Here's how the part is built. I have some questions about the finished solid (model axes, mm). A direction names the side the tool comes from. Coordinates: 2 decimals unless noted, no trailing zeros. Loops run counter-clockwise (first coordinate to the right, second up) from the corner with the lowest first, then second, coordinate; pieces in that order, holes last. Notation, with made-up numbers: (23, -11.75) -> (46, -11.75) arc R18 ccw to (46, 22.25) -> close; hole circle Ø4 at (44.5, 35.25). An arc over 180 degrees is marked (long way). Answer as a JSON object with one key per item and string values. Group by question number.
Q1. I want a section at B-B on x = -1.75. Write out the boundary of the cut face in (y, z), then the cut area to 3 significant figures.
Q2. I need wall thicknesses on line 1 (Z direction, x = -4, y = -11.5); line 2 (Z direction, x = 7, y = -13.5) (3 decimals); line 3 (Y direction, x = 2.75, z = -12.7). Which ranges of each line are inside material? Lowest first, please.
Q3. Thinking about a two-plate mould opening in Y: for faces 1 (the cylindrical face through (0.13, -13.64, -13.88)), 2 (the flat face through (12.7, 21, -20)), 3 (the flat face through (0, -19.05, -25)), which applies, released by +Y, released by -Y, zero draft, split by the parting line, or undercut?
Q4. I want a section at D-D on y = 27.5. Write out the boundary of the cut face in (x, z).
Q5. I want a section at C-C on z = -45. Write out the boundary of the cut face in (x, y).
Q6. I want a section at A-A on z = -12.7. Write out the boundary of the cut face in (x, y), then the cut area to 3 significant figures.
Q7. On a 3-axis mill with a long thin cutter (end or side, diameter ignored), from which of +Z, -Z, +X, -X, +Y, -Y can I reach the whole of each face in a straight line? I mean faces 4 (the flat face through (-11, 0, -26)), 5 (the flat face through (-9.144, -9, -26)), 6 (the flat face through (0, -9, -47.244)). Say none if no direction works.
Q8. I'm going to push flat-ended pins straight in: pin 1 (12 mm diameter, centred on x = -3.5, y = 38, fed in from -Z); pin 2 (8 mm diameter, centred on x = 3, y = -8, fed in from +Z); pin 3 (5.5 mm diameter, centred on y = -9, z = -18, fed in from -X). Where does each tip first touch, or does it pass through?
```python
from build123d import *

# Parameters (mm, degrees)
BOSS_EXTRUDE1_DEPTH = 12.7
SKETCH2_W           = 18.288
SKETCH2_H           = 43.688
BOSS_EXTRUDE2_DEPTH = 19.05
SKETCH3_R           = 2.5527
CUT_EXTRUDE1_DEPTH  = 22.844
CHAMFER1_SIZE       = 1


with BuildPart() as part:
    # Sketch1 → Boss-Extrude1 (new body, symmetric)
    with BuildSketch(Plane(origin=(0, 0, 0), x_dir=(0, 0, -1), z_dir=(1, 0, 0))):
        Polygon((0, 0), (0, 77.724), (50.8, 5.174081258), (50.8, 0), align=None)
    extrude(amount=BOSS_EXTRUDE1_DEPTH, both=True)

    # Sketch2 → Boss-Extrude2 (add)
    with BuildSketch(Plane.XZ):
        with Locations((0, -25.4)):
            Rectangle(SKETCH2_W, SKETCH2_H)
    extrude(amount=BOSS_EXTRUDE2_DEPTH)

    # Sketch3 → Cut-Extrude1 (cut, through all)
    with BuildSketch(Plane(origin=(9.144, 0, 0), x_dir=(0, 0, -1), z_dir=(1, 0, 0))):
        with Locations((38.1, -11.375365521)):
            Circle(SKETCH3_R)
        with Locations((12.7, -11.375365521)):
            Circle(SKETCH3_R)
    extrude(amount=-CUT_EXTRUDE1_DEPTH, mode=Mode.SUBTRACT)

    # Chamfer1
    chamfer1_edges = [part.edges().sort_by_distance(p)[0] for p in [
        (12.7, 41.449040629, -25.4),
        (9.144, -9.525, -47.244),
        (9.144, -9.525, -3.556),
        (-9.144, -9.525, -3.556),
        (12.7, 38.862, 0),
        (-9.144, -9.525, -47.244),
        (-12.7, 38.862, 0),
        (-12.7, 41.449040629, -25.4),
        (-12.7, 2.587040629, -50.8),
        (12.7, 2.587040629, -50.8),
    ]]
    chamfer(chamfer1_edges, length=CHAMFER1_SIZE)


solid = part.part
```
Result set:
{
 "1": {"outline": "(-19.05, -47.24) -> (0, -47.24) -> (0, -50.8) -> (5.17, -50.8) -> (77.72, 0) -> (0, 0) -> (0, -3.56) -> (-19.05, -3.56) -> close; hole circle Ø5.11 at (-11.38, -38.1); hole circle Ø5.11 at (-11.38, -12.7)", "area": "2,900 mm²"},
 "2": {"line 1": "z = -47.24 to -40.65, -35.55 to -15.25, -10.15 to -3.56", "line 2": "z = -47.244 to -39.515, -36.685 to -14.115, -11.285 to -3.556", "line 3": "y = -19.05 to -13.93, -8.82 to 59.59"},
 "3": {"face 1": "undercut", "face 2": "zero draft", "face 3": "released by -Y"},
 "4": {"outline": "(-12.7, -33.95) -> (-11.7, -35.17) -> (11.7, -35.17) -> (12.7, -33.95) -> (12.7, -1) -> (11.7, 0) -> (-11.7, 0) -> (-12.7, -1) -> close"},
 "5": {"outline": "(-12.7, 0) -> (-9.14, 0) -> (-9.14, -19.05) -> (9.14, -19.05) -> (9.14, 0) -> (12.7, 0) -> (12.7, 11.71) -> (11.7, 13.46) -> (-11.7, 13.46) -> (-12.7, 11.71) -> close"},
 "6": {"outline": "(-12.7, 0) -> (-9.14, 0) -> (-9.14, -8.82) -> (9.14, -8.82) -> (9.14, 0) -> (12.7, 0) -> (12.7, 57.84) -> (11.7, 59.59) -> (-11.7, 59.59) -> (-12.7, 57.84) -> close; (-9.14, -19.05) -> (9.14, -19.05) -> (9.14, -13.93) -> (-9.14, -13.93) -> close", "area": "1,770 mm²"},
 "7": {"face 4": "-Y", "face 5": "+Z, -Z, -X, -Y", "face 6": "-Z, +X, -X, -Y"},
 "8": {"pin 1": "stops at z = -32.02", "pin 2": "stops at z = -3.56", "pin 3": "stops at x = -9.14"}
}
